```python
from build123d import *

# Parameters (mm, degrees)
SKETCH1_R               = 19.939
CIRCLE_EXTRUDE_DEPTH    = 7.62
SKETCH3_W               = 7.62
SKETCH3_H               = 39.878
RECTANGLE_EXTRUDE_DEPTH = 63.5
SKETCH2_R               = 18.034
CRICLE_CUT_DEPTH        = 67.991627245
SKETCH4_OUTSIDE_W       = 103.997
SKETCH4_OUTSIDE_H       = 60.436
SKETCH4_OUTSIDE_W_2     = 61.595
SKETCH4_OUTSIDE_H_2     = 36.068
FRAME_CUT_DEPTH         = 67.991627245
EXTENSION_DEPTH         = 2.54
SKETCH13_W              = 5.08
SKETCH13_H              = 36.068
CUT_EXTRUDE1_DEPTH      = 38.1
SKETCH14_R              = 1.905
BOSS_EXTRUDE3_DEPTH     = 2.54


with BuildPart() as part:
    # Sketch1 → circle extrude (new body)
    with BuildSketch(Plane.XY):
        with Locations(Location((0, 0, 0), (0, 0, 180))):
            Circle(SKETCH1_R)
    extrude(amount=CIRCLE_EXTRUDE_DEPTH)

    # Sketch3 → rectangle extrude (add)
    with BuildSketch(Plane(origin=(0, 0, 0), x_dir=(0, 0, -1), z_dir=(1, 0, 0))):
        with Locations((-3.81, 0)):
            Rectangle(SKETCH3_W, SKETCH3_H)
    extrude(amount=RECTANGLE_EXTRUDE_DEPTH)

    # Sketch2 → cricle cut (cut, through all)
    with BuildSketch(Plane.XY.offset(7.62)):
        Circle(SKETCH2_R)
    extrude(amount=-CRICLE_CUT_DEPTH, mode=Mode.SUBTRACT)

    # Sketch4 outside → frame cut (cut, through all)
    with BuildSketch(Plane.XY.offset(7.62)):
        with Locations((21.7805, 0)):
            Rectangle(SKETCH4_OUTSIDE_W, SKETCH4_OUTSIDE_H)
        with Locations((30.7975, 0)):
            Rectangle(SKETCH4_OUTSIDE_W_2, SKETCH4_OUTSIDE_H_2, mode=Mode.SUBTRACT)
    extrude(amount=-FRAME_CUT_DEPTH, mode=Mode.SUBTRACT)

    # Sketch10 → extension (add)
    with BuildSketch(Plane(origin=(0, 0, 0), x_dir=(-1, 0, 0), z_dir=(0, 0, -1))):
        with BuildLine():
            Line((0, 18.034), (-61.595, 18.034))
            Line((-61.595, 18.034), (-61.595, -18.034))
            Line((-61.595, -18.034), (0, -18.034))
            ThreePointArc((0, -18.034), (-18.034, 0), (0, 18.034))
        make_face()
    extrude(amount=EXTENSION_DEPTH)

    # Sketch13 → Cut-Extrude1 (cut)
    with BuildSketch(Plane(origin=(61.595, 0, 0), x_dir=(0, 0, -1), z_dir=(1, 0, 0))):
        with Locations((-2.54, 0)):
            Rectangle(SKETCH13_W, SKETCH13_H)
    extrude(amount=-CUT_EXTRUDE1_DEPTH, mode=Mode.SUBTRACT)

    # Sketch14 → Boss-Extrude3 (add)
    with BuildSketch(Plane(origin=(23.495, 0, 0), x_dir=(0, 0, -1), z_dir=(1, 0, 0))):
        with Locations((-2.54, 0)):
            Circle(SKETCH14_R)
    extrude(amount=BOSS_EXTRUDE3_DEPTH)


solid = part.part
```
The listing builds one solid part. Answer for the finished solid, in the listing's coordinates (mm). A direction names the side the tool comes from. Give positions to 0.01 mm unless a question says otherwise; leave off trailing zeros. Loops run counter-clockwise (first coordinate to the right, second up) from the corner with the lowest first, then second, coordinate; pieces in that order, holes last. Notation, with made-up numbers: (-40, -21) - (2, -21) arc R28 cw to (2, 16) - close; hole circle Ø8 at (-3, -14). An arc over 180 degrees is marked (long way). Answer as CSV lines item,"result". Start each with the question number.
Item 1: For faces 5 (the face through (61.595, 0, -1)), 6 (the face through (43, 0, 0)), 7 (the face through (23.495, 0.3, 4.8)), determine the directions among +Z, -Z, +X, -X, +Y, -Y from which every point of the face is accessible in a straight line to the end or side of a thin tool.
Item 2: A cutting plane is placed at B-B on z = 2.54. Determine the outline of the cut face in (x, y) (3 decimals), then the cut area to 3 significant figures.
Item 3: Find the intervals of material crossed by line 1 (Z direction, x = 54, y = 16); line 2 (Y direction, x = 14, z = 6); line 3 (Y direction, x = 5, z = 3.75), in increasing order. Write a range as from..to.
Item 4: The mould has two halves that part along Y. Classify faces 1 (the face through (38, 0, -2.54)), 2 (the face through (18.03, -0.4, 2.61)), 3 (the face through (24, -18.034, 6)), 4 (the face through (24.75, -1.16, 4.05)): +Y half, -Y half, draft (parallel to the pull), parting line (faces both ways), or undercut.
Item 5: A cutting plane is placed at D-D on x = 10. Determine the outline of the cut face in (y, z).
Item 6: A cutting plane is placed at C-C on y = 0. Determine the outline of the cut face in (x, z) (3 decimals), then the cut area to 3 significant figures.
Item 7: Each of these flat-tipped pins is pushed along its axis until it touches: pin 1 (4 mm diameter, centred on y = 0, z = 2.5, fed in from +X) (3 decimals); pin 2 (1 mm diameter, centred on x = 31.5, z = 3.5, fed in from +Y). Where does it stop, or does it pass through?
Item 8: A cutting plane is placed at A-A on x = 54. Determine the outline of the cut face in (y, z).
Found:
1,face 5,"+Z, -Z, +X, +Y, -Y"
1,face 6,"+X, +Y, -Y"
1,face 7,"+X"
2,outline,"(0, -18.034) - (23.495, -18.034) - (23.495, -1.905) - (26.035, -1.905) - (26.035, 1.905) - (23.495, 1.905) - (23.495, 18.034) - (0, 18.034) arc R18.034 cw to start"
2,area,"346 mm^2"
3,line 1,"z = -2.54..0, 5.08..7.62"
3,line 2,"y = -18.03..-11.37, 11.37..18.03"
3,line 3,"y = -18.03..-17.33, 17.33..18.03"
4,face 1,"draft"
4,face 2,"undercut"
4,face 3,"-Y half"
4,face 4,"parting line"
5,outline,"(-18.03, -2.54) - (-15.01, -2.54) - (-15.01, 7.62) - (-18.03, 7.62) - close; (15.01, -2.54) - (18.03, -2.54) - (18.03, 7.62) - (15.01, 7.62) - close"
6,outline,"(18.034, -2.54) - (61.595, -2.54) - (61.595, 0) - (23.495, 0) - (23.495, 0.635) - (26.035, 0.635) - (26.035, 4.445) - (23.495, 4.445) - (23.495, 5.08) - (61.595, 5.08) - (61.595, 7.62) - (18.034, 7.62) - close"
6,area,"259 mm^2"
7,pin 1,"stops at x = 26.035"
7,pin 2,"passes through"
8,outline,"(-18.03, -2.54) - (18.03, -2.54) - (18.03, 0) - (-18.03, 0) - close; (-18.03, 5.08) - (18.03, 5.08) - (18.03, 7.62) - (-18.03, 7.62) - close"
